```python
from build123d import *

# Parameters (mm, degrees)
SKETCH1_W               = 406.4
SKETCH1_H               = 508
BOSS_EXTRUDE1_DEPTH     = 3.175
SKETCH2_R               = 14.2875
CUT_EXTRUDE1_DEPTH      = 3.175
SKETCH3_R               = 2.4892
CUT_EXTRUDE2_DEPTH      = 1
CUT_EXTRUDE2_DEPTH_BACK = 4.175
SKETCH4_R               = 2.0193
CUT_EXTRUDE3_DEPTH      = 1
CUT_EXTRUDE3_DEPTH_BACK = 4.175
CUT_EXTRUDE4_REACH      = 5.175
SKETCH5_W               = 124.46
SKETCH5_H               = 508
SKETCH5_W_2             = 205.74


with BuildPart() as part:
    # Sketch1 → Boss-Extrude1 (new body)
    with BuildSketch(Plane(origin=(0, 0, 0), x_dir=(1, 0, 0), z_dir=(0, 1, 0))):
        with Locations((203.2, 254)):
            Rectangle(SKETCH1_W, SKETCH1_H)
    extrude(amount=BOSS_EXTRUDE1_DEPTH)

    # Sketch2 → Cut-Extrude1 (cut)
    with BuildSketch(Plane(origin=(0, 3.175, 0), x_dir=(1, 0, 0), z_dir=(0, 1, 0))):
        with Locations((50.8, 419.1)):
            Circle(SKETCH2_R)
        with Locations((165.1, 419.1)):
            Circle(SKETCH2_R)
        with Locations((50.8, 88.9)):
            Circle(SKETCH2_R)
        with Locations((165.1, 88.9)):
            Circle(SKETCH2_R)
    extrude(amount=-CUT_EXTRUDE1_DEPTH, mode=Mode.SUBTRACT)

    # Sketch3 → Cut-Extrude2 (cut, two sides)
    with BuildSketch(Plane(origin=(0, 3.175, 0), x_dir=(1, 0, 0), z_dir=(0, 1, 0))) as cut_extrude2_sk:
        with Locations((38.1, 12.7)):
            Circle(SKETCH3_R)
        with Locations((63.5, 12.7)):
            Circle(SKETCH3_R)
        with Locations((152.4, 12.7)):
            Circle(SKETCH3_R)
        with Locations((177.8, 12.7)):
            Circle(SKETCH3_R)
        with Locations((203.2, 12.7)):
            Circle(SKETCH3_R)
        with Locations((228.6, 12.7)):
            Circle(SKETCH3_R)
        with Locations((254, 12.7)):
            Circle(SKETCH3_R)
        with Locations((279.4, 12.7)):
            Circle(SKETCH3_R)
        with Locations((304.8, 12.7)):
            Circle(SKETCH3_R)
        with Locations((330.2, 12.7)):
            Circle(SKETCH3_R)
        with Locations((355.6, 12.7)):
            Circle(SKETCH3_R)
        with Locations((381, 12.7)):
            Circle(SKETCH3_R)
        with Locations((381, 495.3)):
            Circle(SKETCH3_R)
        with Locations((355.6, 495.3)):
            Circle(SKETCH3_R)
        with Locations((330.2, 495.3)):
            Circle(SKETCH3_R)
        with Locations((304.8, 495.3)):
            Circle(SKETCH3_R)
        with Locations((279.4, 495.3)):
            Circle(SKETCH3_R)
        with Locations((254, 495.3)):
            Circle(SKETCH3_R)
        with Locations((228.6, 495.3)):
            Circle(SKETCH3_R)
        with Locations((203.2, 495.3)):
            Circle(SKETCH3_R)
        with Locations((177.8, 495.3)):
            Circle(SKETCH3_R)
        with Locations((152.4, 495.3)):
            Circle(SKETCH3_R)
        with Locations((63.5, 495.3)):
            Circle(SKETCH3_R)
        with Locations((38.1, 495.3)):
            Circle(SKETCH3_R)
        with Locations((101.6, 12.7)):
            Circle(SKETCH3_R)
    extrude(amount=CUT_EXTRUDE2_DEPTH, mode=Mode.SUBTRACT)
    extrude(cut_extrude2_sk.sketch, amount=-CUT_EXTRUDE2_DEPTH_BACK, mode=Mode.SUBTRACT)

    # Sketch4 → Cut-Extrude3 (cut, two sides)
    with BuildSketch(Plane(origin=(0, 3.175, 0), x_dir=(1, 0, 0), z_dir=(0, 1, 0))) as cut_extrude3_sk:
        with Locations((76.2, 419.1)):
            Circle(SKETCH4_R)
        with Locations((25.4, 419.1)):
            Circle(SKETCH4_R)
        with Locations((38.1, 441.097045256)):
            Circle(SKETCH4_R)
        with Locations((63.5, 441.097045256)):
            Circle(SKETCH4_R)
        with Locations((63.5, 397.102954744)):
            Circle(SKETCH4_R)
        with Locations((38.1, 397.102954744)):
            Circle(SKETCH4_R)
        with Locations((147.139487788, 437.060512212)):
            Circle(SKETCH4_R)
        with Locations((183.060512212, 437.060512212)):
            Circle(SKETCH4_R)
        with Locations((183.060512212, 401.139487788)):
            Circle(SKETCH4_R)
        with Locations((147.139487788, 401.139487788)):
            Circle(SKETCH4_R)
        with Locations((147.139487788, 106.860512212)):
            Circle(SKETCH4_R)
        with Locations((183.060512212, 106.860512212)):
            Circle(SKETCH4_R)
        with Locations((183.060512212, 70.939487788)):
            Circle(SKETCH4_R)
        with Locations((147.139487788, 70.939487788)):
            Circle(SKETCH4_R)
        with Locations((38.1, 110.897045256)):
            Circle(SKETCH4_R)
        with Locations((63.5, 110.897045256)):
            Circle(SKETCH4_R)
        with Locations((63.5, 66.902954744)):
            Circle(SKETCH4_R)
        with Locations((38.1, 66.902954744)):
            Circle(SKETCH4_R)
        with Locations((25.4, 88.9)):
            Circle(SKETCH4_R)
        with Locations((76.2, 88.9)):
            Circle(SKETCH4_R)
    extrude(amount=CUT_EXTRUDE3_DEPTH, mode=Mode.SUBTRACT)
    extrude(cut_extrude3_sk.sketch, amount=-CUT_EXTRUDE3_DEPTH_BACK, mode=Mode.SUBTRACT)

    # Sketch5 → Cut-Extrude4 (cut, up to next)
    with BuildSketch(Plane(origin=(0, 3.175, 0), x_dir=(1, 0, 0), z_dir=(0, 1, 0)), mode=Mode.PRIVATE) as cut_extrude4_sk1:
        with Locations((62.23, 254)):
            Rectangle(SKETCH5_W, SKETCH5_H)
    cut_extrude4_tool1 = extrude(cut_extrude4_sk1.sketch, amount=-CUT_EXTRUDE4_REACH, mode=Mode.PRIVATE) & part.part
    add(cut_extrude4_tool1.solids().sort_by_distance((62.23, 3.175, -254))[0], mode=Mode.SUBTRACT)
    # Sketch5 → Cut-Extrude4 (cut, up to next)
    with BuildSketch(Plane(origin=(0, 3.175, 0), x_dir=(1, 0, 0), z_dir=(0, 1, 0)), mode=Mode.PRIVATE) as cut_extrude4_sk2:
        with Locations((303.53, 254)):
            Rectangle(SKETCH5_W_2, SKETCH5_H)
    cut_extrude4_tool2 = extrude(cut_extrude4_sk2.sketch, amount=-CUT_EXTRUDE4_REACH, mode=Mode.PRIVATE) & part.part
    add(cut_extrude4_tool2.solids().sort_by_distance((303.53, 3.175, -254))[0], mode=Mode.SUBTRACT)


solid = part.part
```
Can you work these out from the model? Positions are in its coordinate system, mm. Give positions to 0.01 mm unless a question says otherwise; leave off trailing zeros. Write each loop counter-clockwise with the first axis right and the second up, starting at its lowest first coordinate (ties: lowest second). Pieces come first, ordered by that corner, then holes. Notation, with made-up numbers: (21, 67) - (63, 67) arc R24 cw to (63, 89) - close; hole circle Ø9 at (4.5, -28). An arc over 180 degrees is marked (long way). Write item = value, one per line. Start each with the question number.
1. Imagine slicing it at A-A (z = -88.9). Please give me the cut outline in (x, y) (1 decimal), and give its area (3 significant figures).
2. Thinking about a two-plate mould opening in X: for faces 1 (the face through (172.78, 1.61, -431.15)), 2 (the face through (178.3, 1.61, -83.43)), 3 (the face through (162, 0, -258)), which applies, released by +X, released by -X, zero draft, split by the parting line, or undercut?
3. Imagine slicing it at B-B (x = 159). Please give me the cut outline in (y, z) (3 decimals), and give its area (3 significant figures).
4. Please list where these lines run through material, in increasing order: line 1 (X direction, y = 2.3, z = -495.3); line 2 (Z direction, x = 183.5, y = 0.6); line 3 (Z direction, x = 176.5, y = 0.35).
5. For pin 1 (4 mm diameter, centred on x = 141, z = -280, fed in from -Y), with a flat end and sliding along its axis, tell me the tip position at first contact or that it passes through.
6. Imagine slicing it at C-C (y = 1.15). Count the separate pieces of the cut face and the enclosed holes in it, and give its area (3 significant figures).
Worked answers:
q1.outline = (124.5, 0) - (150.8, 0) - (150.8, 3.2) - (124.5, 3.2) - close; (179.4, 0) - (200.7, 0) - (200.7, 3.2) - (179.4, 3.2) - close
q1.area = 151 mm2
q2.face_1 = undercut
q2.face_2 = undercut
q2.face_3 = zero draft
q3.outline = (0, -508) - (3.175, -508) - (3.175, -432.02) - (0, -432.02) - close; (0, -406.18) - (3.175, -406.18) - (3.175, -101.82) - (0, -101.82) - close; (0, -75.98) - (3.175, -75.98) - (3.175, 0) - (0, 0) - close
q3.area = 1,450 mm2
q4.line_1 = 124.46 to 149.91, 154.89 to 175.31, 180.29 to 200.66
q4.line_2 = -508 to -439.03, -435.09 to -403.11, -399.17 to -108.83, -104.89 to -72.91, -68.97 to 0
q4.line_3 = -508 to -497.42, -493.18 to -427.71, -410.49 to -97.51, -80.29 to -14.82, -10.58 to 0
q5.pin_1 = 0
q6.separate_pieces = 1
q6.enclosed_holes = 14
q6.area = 37,200 mm2
